Part model, mm, in its own coordinate system. Round coordinates to 2 decimals unless told otherwise and drop trailing zeros. Write each loop counter-clockwise with the first axis right and the second up, starting at its lowest first coordinate (ties: lowest second). Pieces come first, ordered by that corner, then holes.
1) Saw through at A-A on z = -50.8. Write the cut outline in (x, y), and give its area (3 significant figures).
2) Saw through at D-D on x = 137. Write the cut outline in (y, z).
3) Saw through at B-B on x = 95.25. Write the cut outline in (y, z), and give its area (3 significant figures).
4) Drill centre lines: L1, parallel to X at y = 3.25, z = -50.8; L2, parallel to X at y = 2, z = -31.75; L3, parallel to Z at x = 43, y = 0.5. Where is each one in solid material? Low to high.
5) Flat gauge pin, fed straight in: pin 1 (4.5 mm diameter, centred on x = 9.525, z = -12.7, fed in from -Y). Where does the tip first touch, or does it go through?
6) Saw through at C-C on y = 4.5. Count the separate pieces of the cut face and the enclosed holes in it, and give its area (3 significant figures).
```python
from build123d import *

# Parameters (mm, degrees)
SKETCH1_W                    = 190.5
SKETCH1_H                    = 63.5
BOSS_EXTRUDE1_DEPTH          = 6.35
SKETCH3_W                    = 26.9875
SKETCH3_H                    = 26.9875
CUT_EXTRUDE2_DEPTH           = 201.905008648
SKETCH4_W                    = 26.9875
SKETCH4_H                    = 26.9875
CUT_EXTRUDE3_DEPTH           = 201.905008648
SKETCH5_R                    = 15.08125
CUT_EXTRUDE4_DEPTH           = 201.905008648
F_10_0_1935_DIAMETER_HOLE1_D = 4.9149


with BuildPart() as part:
    # Sketch1 → Boss-Extrude1 (new body)
    with BuildSketch(Plane(origin=(0, 0, 0), x_dir=(1, 0, 0), z_dir=(0, 1, 0))):
        with Locations((95.25, 31.75)):
            Rectangle(SKETCH1_W, SKETCH1_H)
    extrude(amount=BOSS_EXTRUDE1_DEPTH)

    # Sketch3 → Cut-Extrude2 (cut, through all)
    with BuildSketch(Plane(origin=(0, 6.35, 0), x_dir=(1, 0, 0), z_dir=(0, 1, 0))):
        with Locations((42.8625, 31.75)):
            Rectangle(SKETCH3_W, SKETCH3_H)
    extrude(amount=-CUT_EXTRUDE2_DEPTH, mode=Mode.SUBTRACT)

    # Sketch4 → Cut-Extrude3 (cut, through all)
    with BuildSketch(Plane(origin=(0, 6.35, 0), x_dir=(1, 0, 0), z_dir=(0, 1, 0))):
        with Locations((147.6375, 31.75)):
            Rectangle(SKETCH4_W, SKETCH4_H)
    extrude(amount=-CUT_EXTRUDE3_DEPTH, mode=Mode.SUBTRACT)

    # Sketch5 → Cut-Extrude4 (cut, through all)
    with BuildSketch(Plane(origin=(0, 6.35, 0), x_dir=(1, 0, 0), z_dir=(0, 1, 0))):
        with Locations(Location((95.25, 31.75, 0), (0, 0, 270))):
            Circle(SKETCH5_R)
    extrude(amount=-CUT_EXTRUDE4_DEPTH, mode=Mode.SUBTRACT)

    # #10 (0.1935) Diameter Hole1 (through all)
    with Locations(Plane(origin=(0, 6.35, 0), x_dir=(1, 0, 0), z_dir=(0, 1, 0))):
        with Locations((9.525, 50.8), (9.525, 12.7), (180.975, 12.7), (180.975, 50.8)):
            Hole(F_10_0_1935_DIAMETER_HOLE1_D / 2)


solid = part.part
```
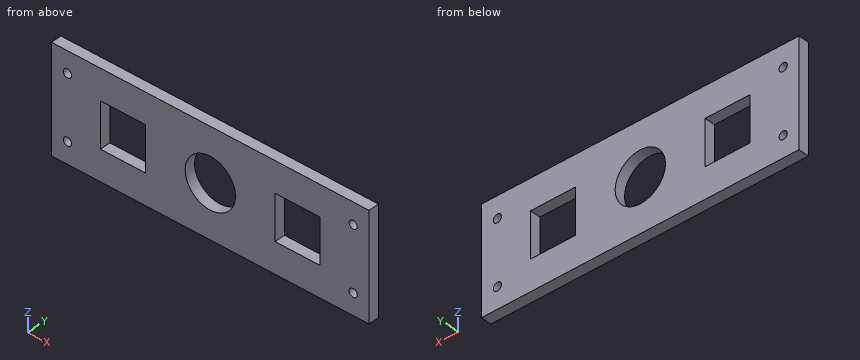
Completed:
1. outline: (0, 0) - (7.07, 0) - (7.07, 6.35) - (0, 6.35) - close; (11.98, 0) - (178.52, 0) - (178.52, 6.35) - (11.98, 6.35) - close; (183.43, 0) - (190.5, 0) - (190.5, 6.35) - (183.43, 6.35) - close
1. area: 1,150 mm2
2. outline: (0, -63.5) - (6.35, -63.5) - (6.35, -45.24) - (0, -45.24) - close; (0, -18.26) - (6.35, -18.26) - (6.35, 0) - (0, 0) - close
3. outline: (0, -63.5) - (6.35, -63.5) - (6.35, -46.83) - (0, -46.83) - close; (0, -16.67) - (6.35, -16.67) - (6.35, 0) - (0, 0) - close
3. area: 212 mm2
4. L1: x = 0 to 7.07, 11.98 to 178.52, 183.43 to 190.5
4. L2: x = 0 to 29.37, 56.36 to 80.17, 110.33 to 134.14, 161.13 to 190.5
4. L3: z = -63.5 to -45.24, -18.26 to 0
5. pin 1: passes through
6. separate pieces: 1
6. enclosed holes: 7
6. area: 9,850 mm2
